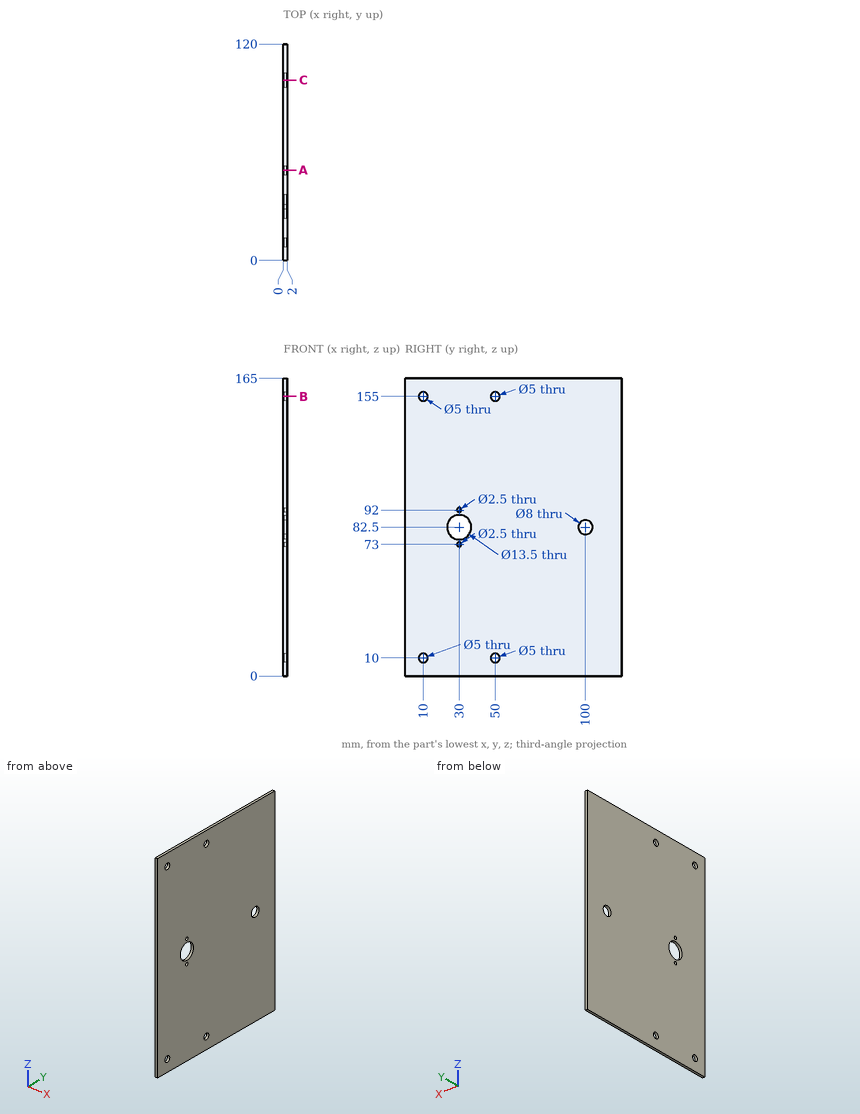
Input: dimensioned drawing with shaded views. Units: mm. Origin: part minimum x, y, z. Coordinates: 2 decimals unless noted, no trailing zeros. Order: outer loops, then holes, each group sorted by start corner. A loop starts at its lowest first (then second) coordinate and runs counter-clockwise, first axis right, second up.
(1) Section query B-B (z = 155). Return the cut outline in (x, y).
(2) First-contact query: pin 1 (3 mm diameter, centred on y = 10, z = 155, fed in from +X). Flat tip, straight axial feed; report the tip coordinate or a pass-through.
(3) Section query C-C (y = 100). Return the cut outline in (x, z), plus the area to 3 significant figures.
(4) Material intervals for probe 1 along Y at (x, z) = (1.5, 82.5); probe 2 along Y at (x, z) = (0.9, 92); probe 3 along Z at (x, y) = (1.5, 30.5), sorted ascending.
(5) Section query A-A (y = 50). Return the cut outline in (x, z), plus the area to 3 significant figures.
Solution:
1. outline: (0, 0) - (2, 0) - (2, 7.5) - (0, 7.5) - close; (0, 12.5) - (2, 12.5) - (2, 47.5) - (0, 47.5) - close; (0, 52.5) - (2, 52.5) - (2, 120) - (0, 120) - close
2. pin 1: passes through
3. outline: (0, 0) - (2, 0) - (2, 78.5) - (0, 78.5) - close; (0, 86.5) - (2, 86.5) - (2, 165) - (0, 165) - close
3. area: 314 mm2
4. probe 1: y = 0 to 23.25, 36.75 to 96, 104 to 120
4. probe 2: y = 0 to 28.75, 31.25 to 120
4. probe 3: z = 0 to 71.85, 74.15 to 75.77, 89.23 to 90.85, 93.15 to 165
5. outline: (0, 0) - (2, 0) - (2, 7.5) - (0, 7.5) - close; (0, 12.5) - (2, 12.5) - (2, 152.5) - (0, 152.5) - close; (0, 157.5) - (2, 157.5) - (2, 165) - (0, 165) - close
5. area: 310 mm2
